Part model, mm, in its own coordinate system. A direction names the side the tool comes from. Round coordinates to 2 decimals unless told otherwise and drop trailing zeros. Loops run counter-clockwise (first coordinate to the right, second up) from the corner with the lowest first, then second, coordinate; pieces in that order, holes last. Notation, with made-up numbers: M 75.25,44.5 L 121.25,44.5 A25 ccw 121.25,61.5 Z; hole C 18.25,57 d6. An arc over 180 degrees is marked long. Put each result on its own line as item: value. Start each with the question number.
1) Drop flat-ended pins along their axis: pin 1 Ø3 at (x, z) = (12, 53) entering from -Y; pin 2 Ø7.5 at (x, y) = (6.5, 126.5) entering from +Z; pin 3 Ø14 at (x, z) = (0.5, 51) entering from -Y. Give the stop position or say it passes through.
2) Probe line 1 along X through (y, z) = (38, 9); line 2 along Y through (x, z) = (-4, 29); line 3 along Z through (x, y) = (14, 30). List the from-to ranges inside material, lowest first.
3) Slice it at A-A on x = 0. Give the cut face in (y, z), then the cut area to 3 significant figures.
4) Slice it at B-B on z = 20.32. Give the cut face in (x, y).
5) Slice it at D-D on z = 48. Give the cut face in (x, y).
6) Slice it at C-C on y = 93.98. Give the cut face in (x, z), then the cut area to 3 significant figures.
7) Pull direction X, two halves, no side cores. Call faces 1 (the flat face through (2.54, 67, 30)), 2 (the cylindrical face through (35.045, 2.897, 17.531)), 3 (the flat face through (0.53, 94.23, 53.59)): +X half, -X half, draft (parallel to the pull), parting line (faces both ways), or undercut.
8) Which spindle directions (+Z, -Z, +X, -X, +Y, -Y) get a long thin tool onto all of the face, cutting with end or side? Do faces 4 (the flat face through (25, 39, 35.56)), 5 (the flat face through (38.1, 78, 28)), 6 (the flat face through (-2.54, 9, 31)), 7 (the flat face through (0, 46, 25.4)), 8 (the cylindrical face through (0.533, 85.917, 14.138)). Say none if no direction does.
```python
from build123d import *

# Parameters (mm, degrees)
F1_DEPTH       = 38.1
F3_D           = 15.24
F3_CBORE_D     = 40.64
F3_CBORE_DEPTH = 10.16
F5_DEPTH       = 76.2
F6_R           = 10.16
F7_DEPTH       = 76.2
F9_DEPTH       = 27.94
F10_R          = 10.16


with BuildPart() as f1:
    # F0 (on Right) → F1 (new body, symmetric)
    with BuildSketch(Plane.YZ):
        Polygon((0, 35.56), (0, 0), (111.76, 0), (147.32, 35.56), (147.32, 71.12), (111.76, 71.12), (76.2, 35.56), align=None)
    extrude(amount=F1_DEPTH, both=True)

    # F3 (through all)
    with Locations(Plane.XY.offset(35.56)):
        with Locations((0, 38.1)):
            CounterBoreHole(F3_D / 2, F3_CBORE_D / 2, F3_CBORE_DEPTH)

    # F4 (on face) → F5 (cut)
    with BuildSketch(Plane.XZ):
        Polygon((2.54, 35.56), (0, 35.56), (-2.54, 35.56), (-2.54, 25.4), (2.54, 25.4), align=None)
    extrude(amount=-F5_DEPTH, mode=Mode.SUBTRACT)

    # F6 (on face) → F7 (cut)
    with BuildSketch(Plane.YZ.offset(38.1)):
        with Locations((93.98, 20.32)):
            Circle(F6_R)
    extrude(amount=-F7_DEPTH, mode=Mode.SUBTRACT)

    # F8 (on face) → F9 (cut)
    with BuildSketch(Plane.XY.offset(71.12)):
        with BuildLine():
            Line((22.86, 137.16), (-22.86, 137.16))
            ThreePointArc((-22.86, 137.16), (-30.48, 129.54), (-22.86, 121.92))
            Line((-22.86, 121.92), (22.86, 121.92))
            ThreePointArc((22.86, 121.92), (30.48, 129.54), (22.86, 137.16))
        make_face()
    extrude(amount=-F9_DEPTH, mode=Mode.SUBTRACT)

    # F10
    f10_edges = [f1.edges().sort_by_distance(p)[0] for p in [
        (38.1, 0, 17.78),
        (-38.1, 0, 17.78),
    ]]
    fillet(f10_edges, radius=F10_R)


solid = f1.part
```
Recorded:
1. pin 1: stops at y = 92.14
1. pin 2: stops at z = 43.18
1. pin 3: stops at y = 84.64
2. line 1: x = -38.1 to -7.62, 7.62 to 38.1
2. line 2: y = 0 to 18.18, 58.02 to 88.7, 99.26 to 140.76
2. line 3: z = 0 to 25.4
3. outline: M 0,0 L 30.48,0 L 30.48,25.4 L 0,25.4 Z; M 45.72,0 L 111.76,0 L 147.32,35.56 L 147.32,71.12 L 137.16,71.12 L 137.16,43.18 L 121.92,43.18 L 121.92,71.12 L 111.76,71.12 L 76.2,35.56 L 76.2,25.4 L 45.72,25.4 Z; hole C 93.98,20.32 d20.32
3. area: 4,590 mm2
4. outline: M -38.1,10.16 A10.16 ccw -27.94,0 L 27.94,0 A10.16 ccw 38.1,10.16 L 38.1,83.82 L -38.1,83.82 Z; M -38.1,104.14 L 38.1,104.14 L 38.1,132.08 L -38.1,132.08 Z; hole C 0,38.1 d15.24
5. outline: M -38.1,88.64 L 38.1,88.64 L 38.1,147.32 L -38.1,147.32 Z; hole M -22.86,121.92 L 22.86,121.92 A7.62 ccw 22.86,137.16 L -22.86,137.16 A7.62 ccw Z
6. outline: M -38.1,0 L 38.1,0 L 38.1,10.16 L -38.1,10.16 Z; M -38.1,30.48 L 38.1,30.48 L 38.1,53.34 L -38.1,53.34 Z
6. area: 2,520 mm2
7. face 1: undercut
7. face 2: +X half
7. face 3: draft
8. face 4: +Z, +X, -X, -Y
8. face 5: +Z, -Z, +X, +Y, -Y
8. face 6: +Z, -Y
8. face 7: +Z
8. face 8: +X, -X
